The model under review builds one solid part; all positions refer to its coordinate system, in mm. A direction names the side the tool comes from. Coordinates: 2 decimals unless noted, no trailing zeros. Order: outer loops, then holes, each group sorted by start corner. A loop starts at its lowest first (then second) coordinate and runs counter-clockwise, first axis right, second up. Notation, with made-up numbers: M 1,-7 L 10,-7 A20 ccw 10,27 Z; hole C 74.5,59 d11. An arc over 180 degrees is marked long. One line per item, written item: value.
```python
from build123d import *

# Parameters (mm, degrees)
F0_R     = 10.6
F1_DEPTH = 1
F2_T     = -0.5
F3_R     = 6.985
F4_DEPTH = 25
F5_R     = 10.6
F5_R_2   = 10.1
F6_DEPTH = 1.5


with BuildPart() as f1:
    # F0 (on Top) → F1 (new body)
    with BuildSketch(Plane.XY):
        Circle(F0_R)
    extrude(amount=F1_DEPTH)

    # F2
    f2_openings = [f1.faces().sort_by_distance(p)[0] for p in [
        (0, 0, 1),
    ]]
    offset(amount=F2_T, openings=f2_openings)

    # F3 (on face) → F4 (cut)
    with BuildSketch(Plane.XY.offset(0.5)):
        Circle(F3_R)
    extrude(amount=-F4_DEPTH, mode=Mode.SUBTRACT)

    # F5 (on face) → F6 (join)
    with BuildSketch(Plane.XY.offset(1)):
        Circle(F5_R)
        Circle(F5_R_2, mode=Mode.SUBTRACT)
    extrude(amount=F6_DEPTH)


solid = f1.part
```
(1) Tool access review of faces 1 (the cylindrical face through (-0.909, 6.926, 0.254)), 2 (the flat face through (7, 2, 0.5)): name each direction out of +Z, -Z, +X, -X, +Y, -Y from which nothing blocks a thin tool from reaching the whole face with its end or side.
Geometry results:
face 1: +Z, -Z
face 2: +Z
(2) Insertion check: pin 1 Ø6 at (x, y) = (2.5, 3.5) entering from +Z; pin 2 Ø1 at (y, z) = (-5, 1.5) entering from -X. Each pin has a flat end and moves straight along its axis. Give the tip position at first contact, or say it passes through.
Geometry results:
pin 1: stops at z = 0.5
pin 2: stops at x = -9.6
(3) Mouldability with a two-part tool opening along Y and no side actions: class faces 3 (the cylindrical face through (9.79, -4.06, 1.23)), 4 (the cylindrical face through (9.634, 3.034, 1.486)), 5 (the flat face through (9, -5, 2.5)) as +Y half, -Y half, draft (parallel to the pull), parting line (faces both ways), or undercut.
Geometry results:
face 3: parting line
face 4: undercut
face 5: draft
(4) For L1, parallel to X at y = -0.25, z = 0.35; L2, parallel to Y at x = 0, z = 0.4 (3 decimals); L3, parallel to Z at x = -6.5, y = -3.5, list the stretches that pass through material, from the lowest coordinate up.
Geometry results:
L1: x = -10.6 to -6.98, 6.98 to 10.6
L2: y = -10.6 to -6.985, 6.985 to 10.6
L3: z = 0 to 0.5
(5) We need section A-A, the plane y = 0. State the section outline as (x, z) points (3 decimals), plus the area to 4 significant figures.
Geometry results:
outline: M -10.6,0 L -6.985,0 L -6.985,0.5 L -10.1,0.5 L -10.1,2.5 L -10.6,2.5 Z; M 6.985,0 L 10.6,0 L 10.6,2.5 L 10.1,2.5 L 10.1,0.5 L 6.985,0.5 Z
area: 5.615 mm2
(6) We need section D-D, the plane y = 9.25. State the section outline as (x, z) points.
Geometry results:
outline: M -5.18,0 L 5.18,0 L 5.18,2.5 L 4.06,2.5 L 4.06,0.5 L -4.06,0.5 L -4.06,2.5 L -5.18,2.5 Z
(7) We need section C-C, the plane z = 2.15. State the section outline as (x, y) points, plus the area to 3 significant figures.
Geometry results:
outline: C 0,0 d21.2; hole C 0,0 d20.2
area: 32.5 mm2
